from build123d import *

# Parameters (mm, degrees)
BOSS_EXTRUDE1_DEPTH      = 152.4
BOSS_EXTRUDE1_DEPTH_BACK = 152.4
SKETCH3_R                = 3.5
CUT_EXTRUDE1_DEPTH       = 306.537297232


with BuildPart() as part:
    # Sketch3 → Boss-Extrude1 (new, two sides: drawn at the far end of the back side and taken through both)
    with BuildSketch(Plane.XY.offset(-BOSS_EXTRUDE1_DEPTH_BACK)):
        with BuildLine():
            Line((-4.55, 15), (-4.55, 14.666666667))
            Line((-4.55, 14.666666667), (-4, 14.666666667))
            Line((-4, 14.666666667), (-4, 13))
            Line((-4, 13), (-8.25, 13))
            Line((-8.25, 13), (-8.25, 9.664213562))
            Line((-8.25, 9.664213562), (-4.585786438, 6))
            Line((-4.585786438, 6), (4.585786438, 6))
            Line((4.585786438, 6), (8.25, 9.664213562))
            Line((8.25, 9.664213562), (8.25, 13))
            Line((8.25, 13), (4, 13))
            Line((4, 13), (4, 14.666666667))
            Line((4, 14.666666667), (4.55, 14.666666667))
            Line((4.55, 14.666666667), (4.55, 15))
            Line((4.55, 15), (13, 15))
            ThreePointArc((13, 15), (14.414213562, 14.414213562), (15, 13))
            Line((15, 13), (15, 4.55))
            Line((15, 4.55), (14.666666667, 4.55))
            Line((14.666666667, 4.55), (14.666666667, 4))
            Line((14.666666667, 4), (13, 4))
            Line((13, 4), (13, 8.25))
            Line((13, 8.25), (9.664213562, 8.25))
            Line((9.664213562, 8.25), (6, 4.585786438))
            Line((6, 4.585786438), (6, -4.585786438))
            Line((6, -4.585786438), (9.664213562, -8.25))
            Line((9.664213562, -8.25), (13, -8.25))
            Line((13, -8.25), (13, -4))
            Line((13, -4), (14.666666667, -4))
            Line((14.666666667, -4), (14.666666667, -4.55))
            Line((14.666666667, -4.55), (15, -4.55))
            Line((15, -4.55), (15, -13))
            ThreePointArc((15, -13), (14.414213562, -14.414213562), (13, -15))
            Line((13, -15), (4.55, -15))
            Line((4.55, -15), (4.55, -14.666666667))
            Line((4.55, -14.666666667), (4, -14.666666667))
            Line((4, -14.666666667), (4, -13))
            Line((4, -13), (8.25, -13))
            Line((8.25, -13), (8.25, -9.664213562))
            Line((8.25, -9.664213562), (4.585786438, -6))
            Line((4.585786438, -6), (-4.585786438, -6))
            Line((-4.585786438, -6), (-8.25, -9.664213562))
            Line((-8.25, -9.664213562), (-8.25, -13))
            Line((-8.25, -13), (-4, -13))
            Line((-4, -13), (-4, -14.666666667))
            Line((-4, -14.666666667), (-4.55, -14.666666667))
            Line((-4.55, -14.666666667), (-4.55, -15))
            Line((-4.55, -15), (-13, -15))
            ThreePointArc((-13, -15), (-14.414213562, -14.414213562), (-15, -13))
            Line((-15, -13), (-15, -4.55))
            Line((-15, -4.55), (-14.666666667, -4.55))
            Line((-14.666666667, -4.55), (-14.666666667, -4))
            Line((-14.666666667, -4), (-13, -4))
            Line((-13, -4), (-13, -8.25))
            Line((-13, -8.25), (-9.664213562, -8.25))
            Line((-9.664213562, -8.25), (-6, -4.585786438))
            Line((-6, -4.585786438), (-6, 4.585786438))
            Line((-6, 4.585786438), (-9.664213562, 8.25))
            Line((-9.664213562, 8.25), (-13, 8.25))
            Line((-13, 8.25), (-13, 4))
            Line((-13, 4), (-14.666666667, 4))
            Line((-14.666666667, 4), (-14.666666667, 4.55))
            Line((-14.666666667, 4.55), (-15, 4.55))
            Line((-15, 4.55), (-15, 13))
            ThreePointArc((-15, 13), (-14.414213562, 14.414213562), (-13, 15))
            Line((-13, 15), (-4.55, 15))
        make_face()
        with Locations(Location((0, 0, 0), (0, 0, 180))):
            Circle(SKETCH3_R, mode=Mode.SUBTRACT)
        with BuildLine():
            Line((-13, 9.25), (-10.25, 9.25))
            ThreePointArc((-10.25, 9.25), (-9.542893219, 9.542893219), (-9.25, 10.25))
            Line((-9.25, 10.25), (-9.25, 13))
            ThreePointArc((-9.25, 13), (-9.542893219, 13.707106781), (-10.25, 14))
            Line((-10.25, 14), (-13, 14))
            ThreePointArc((-13, 14), (-13.707106781, 13.707106781), (-14, 13))
            Line((-14, 13), (-14, 10.25))
            ThreePointArc((-14, 10.25), (-13.707106781, 9.542893219), (-13, 9.25))
        make_face(mode=Mode.SUBTRACT)
        with BuildLine():
            Line((9.25, 13), (9.25, 10.25))
            ThreePointArc((9.25, 10.25), (9.542893219, 9.542893219), (10.25, 9.25))
            Line((10.25, 9.25), (13, 9.25))
            ThreePointArc((13, 9.25), (13.707106781, 9.542893219), (14, 10.25))
            Line((14, 10.25), (14, 13))
            ThreePointArc((14, 13), (13.707106781, 13.707106781), (13, 14))
            Line((13, 14), (10.25, 14))
            ThreePointArc((10.25, 14), (9.542893219, 13.707106781), (9.25, 13))
        make_face(mode=Mode.SUBTRACT)
        with BuildLine():
            Line((13, -9.25), (10.25, -9.25))
            ThreePointArc((10.25, -9.25), (9.542893219, -9.542893219), (9.25, -10.25))
            Line((9.25, -10.25), (9.25, -13))
            ThreePointArc((9.25, -13), (9.542893219, -13.707106781), (10.25, -14))
            Line((10.25, -14), (13, -14))
            ThreePointArc((13, -14), (13.707106781, -13.707106781), (14, -13))
            Line((14, -13), (14, -10.25))
            ThreePointArc((14, -10.25), (13.707106781, -9.542893219), (13, -9.25))
        make_face(mode=Mode.SUBTRACT)
        with BuildLine():
            Line((-9.25, -13), (-9.25, -10.25))
            ThreePointArc((-9.25, -10.25), (-9.542893219, -9.542893219), (-10.25, -9.25))
            Line((-10.25, -9.25), (-13, -9.25))
            ThreePointArc((-13, -9.25), (-13.707106781, -9.542893219), (-14, -10.25))
            Line((-14, -10.25), (-14, -13))
            ThreePointArc((-14, -13), (-13.707106781, -13.707106781), (-13, -14))
            Line((-13, -14), (-10.25, -14))
            ThreePointArc((-10.25, -14), (-9.542893219, -13.707106781), (-9.25, -13))
        make_face(mode=Mode.SUBTRACT)
    extrude(amount=BOSS_EXTRUDE1_DEPTH + BOSS_EXTRUDE1_DEPTH_BACK)

    # Sketch4 → Cut-Extrude1 (cut, through all)
    with BuildSketch(Plane.XY.offset(152.4)):
        Polygon((-0.535555503, 6), (0, 5.625), (0.535555503, 6), align=None)
        Polygon((6, 0.535555503), (5.625, 0), (6, -0.535555503), align=None)
        Polygon((0.535555503, -6), (0, -5.625), (-0.535555503, -6), align=None)
        Polygon((-6, -0.535555503), (-5.625, 0), (-6, 0.535555503), align=None)
        with BuildLine():
            Line((-4.493028589, 3.078815026), (-3.078815026, 1.664601464))
            ThreePointArc((-3.078815026, 1.664601464), (-2.474873734, 2.474873734), (-1.664601464, 3.078815026))
            Line((-1.664601464, 3.078815026), (-3.078815026, 4.493028589))
            Line((-3.078815026, 4.493028589), (-4.493028589, 3.078815026))
        make_face()
        with BuildLine():
            Line((3.078815026, 4.493028589), (1.664601464, 3.078815026))
            ThreePointArc((1.664601464, 3.078815026), (2.474873734, 2.474873734), (3.078815026, 1.664601464))
            Line((3.078815026, 1.664601464), (4.493028589, 3.078815026))
            Line((4.493028589, 3.078815026), (3.078815026, 4.493028589))
        make_face()
        with BuildLine():
            Line((4.493028589, -3.078815026), (3.078815026, -1.664601464))
            ThreePointArc((3.078815026, -1.664601464), (2.474873734, -2.474873734), (1.664601464, -3.078815026))
            Line((1.664601464, -3.078815026), (3.078815026, -4.493028589))
            Line((3.078815026, -4.493028589), (4.493028589, -3.078815026))
        make_face()
        with BuildLine():
            Line((-3.078815026, -4.493028589), (-1.664601464, -3.078815026))
            ThreePointArc((-1.664601464, -3.078815026), (-2.474873734, -2.474873734), (-3.078815026, -1.664601464))
            Line((-3.078815026, -1.664601464), (-4.493028589, -3.078815026))
            Line((-4.493028589, -3.078815026), (-3.078815026, -4.493028589))
        make_face()
    extrude(amount=-CUT_EXTRUDE1_DEPTH, mode=Mode.SUBTRACT)


solid = part.part
Can you work these out from the model? Positions are in its coordinate system, mm. Coordinates: 2 decimals unless noted, no trailing zeros. Answer as a JSON object with one key per item and string values. Group by question number.
Item 1: If we mould it in two halves opening along X, with no side actions, what happens to faces 1 (the face through (9, 15, -2)), 2 (the face through (-15, -9, -2)), 3 (the face through (15, -9, -2))? For each: released by +X, released by -X, zero draft, split by the parting line, or undercut.
Item 2: If I drill on L1, parallel to Y at x = -10.5, z = 94; L2, parallel to Y at x = -8, z = 14.5, over which ranges is the centre line in solid material (lowest first)? Write a range as from..to.
Item 3: For pin 1 (3 mm diameter, centred on x = 3, z = 41.5, fed in from -Y); pin 2 (1.8 mm diameter, centred on y = -14, z = 31, fed in from -X); pin 3 (2 mm diameter, centred on x = -2, z = -17, fed in from -Y), each with a flat end and sliding along its axis, tell me the tip position at first contact or that it passes through.
Item 4: If we section it at A-A (z = -110.5): State how many separate pieces and enclosed holes the cut face has, plus the area to 3 significant figures.
Returned:
{
 "1": {"face 1": "zero draft", "face 2": "released by -X", "face 3": "released by +X"},
 "2": {"L1": "y = -15..-14, -9.25..-8.25, 8.25..9.25, 14..15", "L2": "y = -15..-13, -9.41..-6.59, 6.59..9.41, 13..15"},
 "3": {"pin 1": "stops at y = -14.67", "pin 2": "stops at x = -15", "pin 3": "stops at y = -6"},
 "4": {"separate pieces": "1", "enclosed holes": "5", "area": "281 mm²"}
}
